Could you check a few things on this model? Use its own coordinates, in mm. Face numbers are marked on the shaded views. A direction names the side the tool comes from. Round coordinates to 2 decimals unless told otherwise and drop trailing zeros. Write each loop counter-clockwise with the first axis right and the second up, starting at its lowest first coordinate (ties: lowest second). Pieces come first, ordered by that corner, then holes. Notation, with made-up numbers: (87, 75.25) -> (134, 75.25) arc R27 cw to (134, 106.25) -> close; hole circle Ø7 at (60, 64). An arc over 180 degrees is marked (long way). Answer in a Markdown table with one row per item.
from build123d import *

# Parameters (mm, degrees)
SKETCH1_W           = 10
SKETCH1_H           = 37
BOSS_EXTRUDE1_DEPTH = 2
SKETCH2_W           = 10
SKETCH2_H           = 10
SKETCH2_R           = 3.4
BOSS_EXTRUDE2_DEPTH = 4
SKETCH3_R           = 1.6
CUT_EXTRUDE1_DEPTH  = 2
FILLET1_R           = 3.5
SKETCH4_R           = 1.5
CUT_EXTRUDE2_DEPTH  = 2


with BuildPart() as part:
    # Sketch1 → Boss-Extrude1 (new body)
    with BuildSketch(Plane.XY):
        with Locations((-12.863567867, 10.18847884)):
            Rectangle(SKETCH1_W, SKETCH1_H)
    extrude(amount=BOSS_EXTRUDE1_DEPTH)

    # Sketch2 → Boss-Extrude2 (add)
    with BuildSketch(Plane.XY.offset(2)):
        with Locations((-12.863567867, -3.31152116)):
            Rectangle(SKETCH2_W, SKETCH2_H)
        with Locations((-12.863567867, -3.31152116)):
            Circle(SKETCH2_R, mode=Mode.SUBTRACT)
    extrude(amount=BOSS_EXTRUDE2_DEPTH)

    # Sketch3 → Cut-Extrude1 (cut)
    with BuildSketch(Plane.XY.offset(2)):
        with Locations((-12.863567867, 25.68847884)):
            Circle(SKETCH3_R)
    extrude(amount=-CUT_EXTRUDE1_DEPTH, mode=Mode.SUBTRACT)

    # Fillet1
    fillet1_edges = [part.edges().sort_by_distance(p)[0] for p in [
        (-7.863567867, -8.31152116, 3),
        (-17.863567867, -8.31152116, 3),
        (-17.863567867, 1.68847884, 4),
        (-7.863567867, 1.68847884, 4),
    ]]
    fillet(fillet1_edges, radius=FILLET1_R)

    # Sketch4 → Cut-Extrude2 (cut)
    with BuildSketch(Plane.XY.offset(2)):
        with Locations((-12.863567867, -3.31152116)):
            Circle(SKETCH4_R)
    extrude(amount=-CUT_EXTRUDE2_DEPTH, mode=Mode.SUBTRACT)


solid = part.part
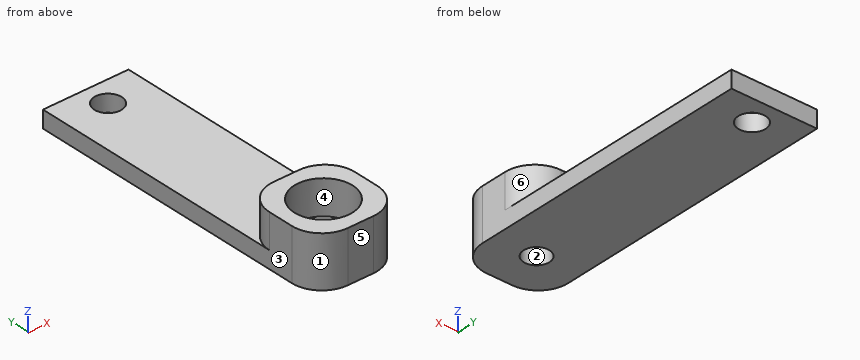
1) For pin 1 (2 mm diameter, centred on x = -10, z = 4, fed in from +Y); pin 2 (5 mm diameter, centred on x = -12.86, y = -3.31, fed in from +Z), each with a flat end and sliding along its axis, tell me the tip position at first contact or that it passes through.
Findings:
| item | result |
|---|---|
| pin 1 | stops at y = 1.67 |
| pin 2 | stops at z = 2 |
2) Please list where these lines run through material, in increasing order: line 1 (Y direction, x = -13.5, z = 1.55); line 2 (Z direction, x = -10.5, y = 25); line 3 (Y direction, x = -11.5, z = 1.5).
Findings:
| item | result |
|---|---|
| line 1 | y = -8.31 to -4.67, -1.95 to 24.22, 27.16 to 28.69 |
| line 2 | z = 0 to 2 |
| line 3 | y = -8.31 to -3.94, -2.69 to 24.85, 26.53 to 28.69 |
3) Imagine slicing it at A-A, the plane x = -12. Please give me the cut outline in (y, z), plus the area to 3 significant figures.
Findings:
| item | result |
|---|---|
| outline | (-8.31, 0) -> (-4.54, 0) -> (-4.54, 2) -> (-6.6, 2) -> (-6.6, 6) -> (-8.31, 6) -> close; (-2.09, 0) -> (24.34, 0) -> (24.34, 2) -> (1.69, 2) -> (1.69, 6) -> (-0.02, 6) -> (-0.02, 2) -> (-2.09, 2) -> close; (27.04, 0) -> (28.69, 0) -> (28.69, 2) -> (27.04, 2) -> close |
| area | 77.4 mm^2 |
4) For the marked faces 4, 5 and 6, which set-ups out of +Z, -Z, +X, -X, +Y, -Y let a thin tool reach every point of the face, with its end or its side?
Findings:
| item | result |
|---|---|
| face 4 | +Z |
| face 5 | +Z, -Z, +X, -X, -Y |
| face 6 | +Z, +X, +Y |
5) Imagine slicing it at B-B, the plane z = 4.2. Please give me the cut outline in (x, y).
Findings:
| item | result |
|---|---|
| outline | (-17.86, -4.81) arc R3.5 ccw to (-14.36, -8.31) -> (-11.36, -8.31) arc R3.5 ccw to (-7.86, -4.81) -> (-7.86, -1.81) arc R3.5 ccw to (-11.36, 1.69) -> (-14.36, 1.69) arc R3.5 ccw to (-17.86, -1.81) -> close; hole circle Ø6.8 at (-12.86, -3.31) |
6) Imagine slicing it at D-D, the plane z = 1.3. Please give me the cut outline in (x, y).
Findings:
| item | result |
|---|---|
| outline | (-17.86, -4.81) arc R3.5 ccw to (-14.36, -8.31) -> (-11.36, -8.31) arc R3.5 ccw to (-7.86, -4.81) -> (-7.86, 28.69) -> (-17.86, 28.69) -> close; hole circle Ø3.2 at (-12.86, 25.69); hole circle Ø3 at (-12.86, -3.31) |
7) Thinking about a two-plate mould opening in Y: for the marked faces 1, 2 and 3, which applies, +Y half, -Y half, draft (parallel to the pull), parting line (faces both ways), or undercut?
Findings:
| item | result |
|---|---|
| face 1 | -Y half |
| face 2 | undercut |
| face 3 | draft |
8) Imagine slicing it at C-C, the plane y = -5.5. Please give me the cut outline in (x, z), plus the area to 3 significant figures.
Findings:
| item | result |
|---|---|
| outline | (-17.8, 0) -> (-7.93, 0) -> (-7.93, 6) -> (-10.26, 6) -> (-10.26, 2) -> (-15.47, 2) -> (-15.47, 6) -> (-17.8, 6) -> close |
| area | 38.4 mm^2 |
